from build123d import *

# Parameters (mm, degrees)
F0_R     = 30
F1_DEPTH = 7
F3_R     = 7.5
F4_DEPTH = 25
F5_R     = 2
F6_R     = 2


with BuildPart() as f1:
    # F0 (on Top) → F1 (new body)
    with BuildSketch(Plane.XY):
        Circle(F0_R)
    extrude(amount=F1_DEPTH)

    # F3 (on face) → F4 (cut)
    with BuildSketch(Plane.XY.offset(7)):
        Circle(F3_R)
    extrude(amount=-F4_DEPTH, mode=Mode.SUBTRACT)

    # F5
    f5_edges = [f1.edges().sort_by_distance(p)[0] for p in [
        (-7.5, 0, 7),
        (-7.5, 0, 0),
    ]]
    fillet(f5_edges, radius=F5_R)

    # F6
    f6_edges = [f1.edges().sort_by_distance(p)[0] for p in [
        (-30, 0, 7),
        (-30, 0, 0),
    ]]
    fillet(f6_edges, radius=F6_R)


solid = f1.part
Here's how the part is built. I have some questions about the finished solid (model axes, mm). Give positions to 0.01 mm unless a question says otherwise; leave off trailing zeros. Loops run counter-clockwise (first coordinate to the right, second up) from the corner with the lowest first, then second, coordinate; pieces in that order, holes last. Notation, with made-up numbers: (46.5, -5) -> (93.5, -5) arc R10 cw to (93.5, 14) -> close; hole circle Ø2 at (27, -33). An arc over 180 degrees is marked (long way). Answer as a JSON object with one key per item and string values. Group by question number.
Item 1: Thinking about a two-plate mould opening in X: for faces 1 (the cylindrical face through (-29.97, 1.32, 3.48)), 2 (the flat face through (0, -12, 7)), 3 (the cylindrical face through (-7.493, 0.33, 3.521)), which applies, pulls with the +X half, pulls with the -X half, needs draft (parallel to the pull), parting line crosses it, or undercut?
Item 2: I need wall thicknesses on L1, parallel to Y at x = 0, z = 4.35; L2, parallel to Z at x = 7.5, y = 5.5; L3, parallel to Y at x = 0.5, z = 1. Which ranges of each line are inside material? Lowest first, please.
Item 3: Imagine slicing it at A-A on x = 0. Write out the boundary of the cut face in (y, z).
Item 4: Imagine slicing it at C-C on z = 3.5. Write out the boundary of the cut face in (x, y), then the cut area to 3 significant figures.
Item 5: Will these pins go through, and if not, where does the flat tip stop? pin 1 (3 mm diameter, centred on y = -14, z = 1, fed in from +X); pin 2 (3 mm diameter, centred on y = -13, z = 5, fed in from -X); pin 3 (2 mm diameter, centred on x = -23, z = 1.5, fed in from +Y); pin 4 (12 mm diameter, centred on x = 0, y = 0, fed in from -Z).
Answer list:
{
 "1": {"face 1": "parting line crosses it", "face 2": "needs draft", "face 3": "undercut"},
 "2": {"L1": "y = -30 to -7.5, 7.5 to 30", "L2": "z = 0.01 to 6.99", "L3": "y = -29.73 to -7.75, 7.75 to 29.73"},
 "3": {"outline": "(-30, 2) arc R2 ccw to (-28, 0) -> (-9.5, 0) arc R2 ccw to (-7.5, 2) -> (-7.5, 5) arc R2 ccw to (-9.5, 7) -> (-28, 7) arc R2 ccw to (-30, 5) -> close; (7.5, 2) arc R2 ccw to (9.5, 0) -> (28, 0) arc R2 ccw to (30, 2) -> (30, 5) arc R2 ccw to (28, 7) -> (9.5, 7) arc R2 ccw to (7.5, 5) -> close"},
 "4": {"outline": "circle Ø60 at (0, 0); hole circle Ø15 at (0, 0)", "area": "2,650 mm2"},
 "5": {"pin 1": "stops at x = 27.17", "pin 2": "stops at x = -27.71", "pin 3": "stops at y = 20.34", "pin 4": "passes through"}
}
